```python
from build123d import *

# Parameters (mm, degrees)
F1_DEPTH = 5
F2_R     = 4
F4_D     = 3.3
F5_W     = 18
F5_H     = 18
F6_DEPTH = 5.001
F8_D     = 3.3


with BuildPart() as f1:
    # F0 (on Top) → F1 (new body)
    with BuildSketch(Plane.XY):
        with BuildLine():
            Line((12.5, 37.5), (-12.5, 37.5))
            ThreePointArc((-12.5, 37.5), (-30.1776695297, 30.1776695297), (-37.5, 12.5))
            Line((-37.5, 12.5), (-37.5, -12.5))
            ThreePointArc((-37.5, -12.5), (-30.1776695297, -30.1776695297), (-12.5, -37.5))
            Line((-12.5, -37.5), (12.5, -37.5))
            ThreePointArc((12.5, -37.5), (30.1776695297, -30.1776695297), (37.5, -12.5))
            Line((37.5, -12.5), (37.5, 12.5))
            ThreePointArc((37.5, 12.5), (30.1776695297, 30.1776695297), (12.5, 37.5))
        make_face()
    extrude(amount=F1_DEPTH)

    # F2
    f2_edges = [f1.edges().sort_by_distance(p)[0] for p in [
        (37.5, 0, 5),
        (30.17767, 30.17767, 5),
        (0, 37.5, 5),
        (-30.17767, 30.17767, 5),
        (-37.5, 0, 5),
        (-30.17767, -30.17767, 5),
        (0, -37.5, 5),
        (30.17767, -30.17767, 5),
    ]]
    fillet(f2_edges, radius=F2_R)

    # F4 (through all)
    with Locations(Plane.XY.offset(5)):
        with Locations((-28, 18.5), (28, 18.5), (-13.5, -31), (13.5, -31)):
            Hole(F4_D / 2)

    # F5 (on face) → F6 (cut, through all)
    with BuildSketch(Plane.XY.offset(5)):
        with Locations((0, -28.5)):
            Rectangle(F5_W, F5_H)
    extrude(amount=-F6_DEPTH, mode=Mode.SUBTRACT)

    # F8 (through all)
    with Locations(Plane.XY.offset(5)):
        with Locations((-15, 28), (15, 28)):
            Hole(F8_D / 2)


solid = f1.part
```
Check sheet for the modelled part. Datum: model origin and axes. Units: mm. A direction names the side the tool comes from. Give positions to 0.01 mm unless a question says otherwise; leave off trailing zeros. Write each loop counter-clockwise with the first axis right and the second up, starting at its lowest first coordinate (ties: lowest second). Pieces come first, ordered by that corner, then holes.
Item 1: Draft check along Y on faces 1 (the face through (14.11, 29.39, 2.47)), 2 (the face through (-10.726, -36.359, 3.797)), 3 (the face through (30.371, 29.982, 0.493)). Enter one of: released by +Y, released by -Y, zero draft, split by the parting line, or undercut.
Item 2: Scan lines: L1, parallel to Y at x = -13.5, z = 1.55; L2, parallel to Y at x = -13.5, z = 2.2; L3, parallel to Y at x = -28, z = 1.75. Record each from-to range of solid material in increasing order.
Item 3: Cross-section at A-A (z = 2.3). Enter the section's corners in (x, y), and give its area (3 significant figures).
Item 4: Cross-section at D-D (x = 1). Enter the section's corners in (y, z).
Item 5: Gauge pin test, flat ends, axial feed: pin 1 (1.5 mm diameter, centred on y = -31, z = 2.5, fed in from +X); pin 2 (1 mm diameter, centred on x = 28, z = 2, fed in from +Y); pin 3 (1.5 mm diameter, centred on x = 4, z = 2.5, fed in from +Y); pin 4 (3 mm diameter, centred on x = -28, y = 18.5, fed in from -Z). Record the tip position at first contact, or that the pin passes through.
Item 6: Cross-section at B-B (x = 11). Enter the section's corners in (y, z).
Item 7: Cross-section at C-C (y = 28). Count the separate pieces of the cut face and the enclosed holes in it, and give its area (3 significant figures).
Item 8: Access from +Z, -Z, +X, -X, +Y, -Y to the whole of each face (thin tool, end or side, straight path). Record for faces 4 (the face through (-15.89, 29.39, 2.47)), 5 (the face through (9, -29, 3)).
Report:
1. face 1: undercut
1. face 2: released by -Y
1. face 3: released by +Y
2. L1: y = -37.44 to -32.65, -29.35 to 27.31, 28.69 to 37.44
2. L2: y = -37.3 to -32.65, -29.35 to 27.31, 28.69 to 37.3
2. L3: y = -32.02 to 16.85, 20.15 to 32.02
3. outline: (-37.28, -12.5) arc R24.78 ccw to (-12.5, -37.28) - (-9, -37.28) - (-9, -19.5) - (9, -19.5) - (9, -37.28) - (12.5, -37.28) arc R24.78 ccw to (37.28, -12.5) - (37.28, 12.5) arc R24.78 ccw to (12.5, 37.28) - (-12.5, 37.28) arc R24.78 ccw to (-37.28, 12.5) - close; hole circle Ø3.3 at (-28, 18.5); hole circle Ø3.3 at (-15, 28); hole circle Ø3.3 at (-13.5, -31); hole circle Ø3.3 at (13.5, -31); hole circle Ø3.3 at (15, 28); hole circle Ø3.3 at (28, 18.5)
3. area: 4,660 mm2
4. outline: (-19.5, 0) - (37.5, 0) - (37.5, 1) arc R4 ccw to (33.5, 5) - (-19.5, 5) - close
5. pin 1: stops at x = 29.78
5. pin 2: stops at y = 32.37
5. pin 3: stops at y = 37.43
5. pin 4: passes through
6. outline: (-37.5, 0) - (37.5, 0) - (37.5, 1) arc R4 ccw to (33.5, 5) - (-33.5, 5) arc R4 ccw to (-37.5, 1) - close
7. separate pieces: 3
7. enclosed holes: 0
7. area: 279 mm2
8. face 4: +Z, -Z
8. face 5: +Z, -Z, -Y
